```python
from build123d import *

# Parameters (mm, degrees)
CROQUIS1_W                 = 42
CROQUIS1_H                 = 42
SALIENTE_EXTRUIR1_DEPTH    = 6
CROQUIS2_R                 = 15
SALIENTE_EXTRUIR2_DEPTH    = 32
CROQUIS3_W                 = 42
CROQUIS3_H                 = 42
SALIENTE_EXTRUIR3_DEPTH    = 8
CROQUIS4_R                 = 11
CORTAR_EXTRUIR1_DEPTH      = 55.753995288
CROQUIS5_R                 = 1.75
CORTAR_EXTRUIR2_DEPTH      = 10
CHAFL_N1_SIZE              = 4
REDONDEO1_R                = 4
CROQUIS6_R                 = 2.25
CORTAR_EXTRUIR3_DEPTH      = 10
REDONDEO2_R                = 4
CORTAR_EXTRUIR4_DEPTH      = 55.753995288
CORTAR_EXTRUIR4_DEPTH_BACK = 55.753995288


with BuildPart() as part:
    # Croquis1 → Saliente-Extruir1 (new body)
    with BuildSketch(Plane.XY):
        Rectangle(CROQUIS1_W, CROQUIS1_H)
    extrude(amount=SALIENTE_EXTRUIR1_DEPTH)

    # Croquis2 → Saliente-Extruir2 (add)
    with BuildSketch(Plane.XY.offset(6)):
        Circle(CROQUIS2_R)
    extrude(amount=SALIENTE_EXTRUIR2_DEPTH)

    # Croquis3 → Saliente-Extruir3 (add)
    with BuildSketch(Plane.XY.offset(38)):
        Rectangle(CROQUIS3_W, CROQUIS3_H)
    extrude(amount=SALIENTE_EXTRUIR3_DEPTH)

    # Croquis4 → Cortar-Extruir1 (cut, through all)
    with BuildSketch(Plane.XY.offset(46)):
        Circle(CROQUIS4_R)
    extrude(amount=-CORTAR_EXTRUIR1_DEPTH, mode=Mode.SUBTRACT)

    # Croquis5 → Cortar-Extruir2 (cut)
    with BuildSketch(Plane.XY.offset(46)):
        with Locations((15.5, 15.5)):
            Circle(CROQUIS5_R)
        with Locations((-15.5, 15.5)):
            Circle(CROQUIS5_R)
        with Locations((-15.5, -15.5)):
            Circle(CROQUIS5_R)
        with Locations((15.5, -15.5)):
            Circle(CROQUIS5_R)
    extrude(amount=-CORTAR_EXTRUIR2_DEPTH, mode=Mode.SUBTRACT)

    # Chaflán1
    chafl_n1_edges = [part.edges().sort_by_distance(p)[0] for p in [
        (21, -21, 42),
        (21, 21, 42),
        (-21, 21, 42),
        (-21, -21, 42),
    ]]
    chamfer(chafl_n1_edges, length=CHAFL_N1_SIZE)

    # Redondeo1
    redondeo1_edges = [part.edges().sort_by_distance(p)[0] for p in [
        (-15, 0, 6),
        (-15, 0, 38),
    ]]
    fillet(redondeo1_edges, radius=REDONDEO1_R)

    # Croquis6 → Cortar-Extruir3 (cut)
    with BuildSketch(Plane(origin=(0, 0, 0), x_dir=(-1, 0, 0), z_dir=(0, 0, -1))):
        with Locations((17, 17)):
            Circle(CROQUIS6_R)
        with Locations((17, -17)):
            Circle(CROQUIS6_R)
        with Locations((-17, -17)):
            Circle(CROQUIS6_R)
        with Locations((-17, 17)):
            Circle(CROQUIS6_R)
    extrude(amount=-CORTAR_EXTRUIR3_DEPTH, mode=Mode.SUBTRACT)

    # Redondeo2
    redondeo2_edges = [part.edges().sort_by_distance(p)[0] for p in [
        (21, -21, 3),
        (-21, -21, 3),
        (-21, 21, 3),
        (21, 21, 3),
    ]]
    fillet(redondeo2_edges, radius=REDONDEO2_R)

    # Croquis7 → Cortar-Extruir4 (cut, two sides: drawn at the far end of the back side and taken through both)
    with BuildSketch(Plane(origin=(0, 0, 0), x_dir=(0, 0, -1), z_dir=(1, 0, 0)).offset(-CORTAR_EXTRUIR4_DEPTH_BACK)):
        with BuildLine():
            Line((-34, 4), (-10, 4))
            ThreePointArc((-10, 4), (-6, 0), (-10, -4))
            Line((-10, -4), (-34, -4))
            ThreePointArc((-34, -4), (-38, 0), (-34, 4))
        make_face()
    extrude(amount=CORTAR_EXTRUIR4_DEPTH + CORTAR_EXTRUIR4_DEPTH_BACK, mode=Mode.SUBTRACT)


solid = part.part
```
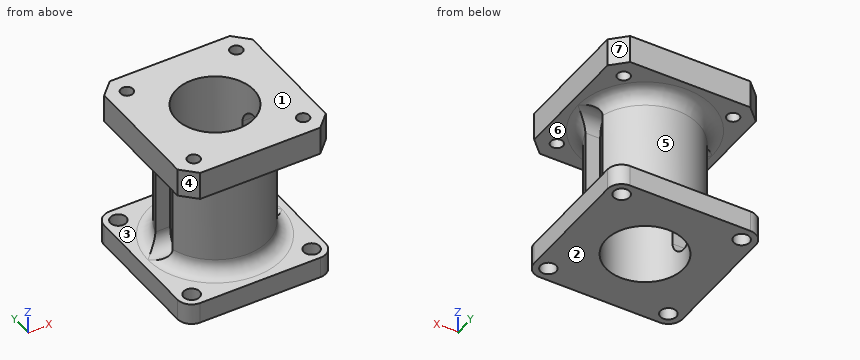
Work out the finished part from the listing and answer in its coordinate system (mm). Face numbers are marked on the shaded views. A direction names the side the tool comes from. Round coordinates to 2 decimals unless told otherwise and drop trailing zeros. Write each loop counter-clockwise with the first axis right and the second up, starting at its lowest first coordinate (ties: lowest second). Pieces come first, ordered by that corner, then holes.
1) A cutting plane is placed at B-B on z = 23. Determine the outline of the cut face in (x, y).
2) Consider probe 1 along Y at (x, z) = (17, 1.65); probe 2 along Y at (x, z) = (-15.5, 43.5); probe 3 along Y at (x, z) = (0, 17.5). Determine where each line is inside the solid, lowest interval first.
3) Which of the six approach directions +Z, -Z, +X, -X, +Y, -Y give full straight-line access (tool end or side, diameter ignored) to the marked faces 5, 6 and 7?
4) A cutting plane is placed at D-D on y = 3. Give the number of separate pieces and of enclosed holes in the cut face, and give its area (3 significant figures).
5) Determine the mould class of the marked faces 1, 2, 3 and 4 for opening direction Z: pulls with the +Z half, pulls with the -Z half, needs draft (parallel to the pull), parting line crosses it, or undercut.
6) A cutting plane is placed at C-C on z = 4.5. Determine the outline of the cut face in (x, y).
7) Flat-ended cylindrical pins translate along their axes: P1, Ø2, axis at x = -15.5, y = 15.5, coming from the -Z side; P2, Ø2, axis at x = -5, y = -7, coming from the -Z side; P3, Ø3.5, axis at x = -11.5, z = 19, coming from the -Y side; P4, Ø4.5, axis at x = -13, z = 17, coming from the +Y side. Find the tip coordinate at first contact, or state that the pin passes through.
8) A cutting plane is placed at A-A on x = 0. Determine the outline of the cut face in (y, z), and give its area (3 significant figures).
Entries:
1. outline: (-14.46, -4) arc R15 ccw to (14.46, -4) - (10.25, -4) arc R11 cw to (-10.25, -4) - close; (-14.46, 4) - (-10.25, 4) arc R11 cw to (10.25, 4) - (14.46, 4) arc R15 ccw to start
2. probe 1: y = -21 to -19.25, -14.75 to 14.75, 19.25 to 21
2. probe 2: y = -21 to -17.25, -13.75 to 13.75, 17.25 to 21
2. probe 3: y = -15 to -11, 11 to 15
3. face 5: +Y
3. face 6: none
3. face 7: +Z, +X, +Y
4. separate pieces: 4
4. enclosed holes: 0
4. area: 325 mm2
5. face 1: pulls with the +Z half
5. face 2: pulls with the -Z half
5. face 3: undercut
5. face 4: needs draft
6. outline: (-21, -17) arc R4 ccw to (-17, -21) - (17, -21) arc R4 ccw to (21, -17) - (21, 17) arc R4 ccw to (17, 21) - (-17, 21) arc R4 ccw to (-21, 17) - close; hole circle Ø4.5 at (-17, -17); hole circle Ø4.5 at (-17, 17); hole circle Ø22 at (0, 0); hole circle Ø4.5 at (17, -17); hole circle Ø4.5 at (17, 17)
7. P1: stops at z = 0
7. P2: passes through
7. P3: stops at y = -11.4
7. P4: stops at y = 10.46
8. outline: (-21, 0) - (-11, 0) - (-11, 46) - (-21, 46) - (-21, 38) - (-19, 38) arc R4 cw to (-15, 34) - (-15, 10) arc R4 cw to (-19, 6) - (-21, 6) - close; (11, 0) - (21, 0) - (21, 6) - (19, 6) arc R4 cw to (15, 10) - (15, 34) arc R4 cw to (19, 38) - (21, 38) - (21, 46) - (11, 46) - close
8. area: 550 mm2
